from build123d import *

# Parameters (mm, degrees)
SKETCH_1_R          = 12.5
SKETCH_1_R_2        = 3
EXTRUDE_1_DEPTH     = 8
SKETCH_2_R          = 2
CUT_EXTRUDE_1_DEPTH = 13.5
SKETCH_3_R          = 1.5
CUT_EXTRUDE_2_DEPTH = 9.0000001


with BuildPart() as part:
    # 草图1 → 凸台-拉伸1 (new body)
    with BuildSketch(Plane.XY):
        Circle(SKETCH_1_R)
        with Locations((0, -6.3)):
            Circle(SKETCH_1_R_2, mode=Mode.SUBTRACT)
    extrude(amount=EXTRUDE_1_DEPTH)

    # 草图2 → 切除-拉伸1 (cut, through all)
    with BuildSketch(Plane(origin=(0, 0, 0), x_dir=(0, 0, -1), z_dir=(1, 0, 0))):
        with Locations((-4, -6.3)):
            Circle(SKETCH_2_R)
    extrude(amount=-CUT_EXTRUDE_1_DEPTH, mode=Mode.SUBTRACT)

    # 草图3 → 切除-拉伸2 (cut, through all)
    with BuildSketch(Plane.XY.offset(8)):
        with Locations((-5, 5)):
            Circle(SKETCH_3_R)
        with Locations((5, 5)):
            Circle(SKETCH_3_R)
    extrude(amount=-CUT_EXTRUDE_2_DEPTH, mode=Mode.SUBTRACT)


solid = part.part
Design review of the part built by this model. Coordinates are the model's own, in mm. A direction names the side the tool comes from. Coordinates: 2 decimals unless noted, no trailing zeros. Order: outer loops, then holes, each group sorted by start corner. A loop starts at its lowest first (then second) coordinate and runs counter-clockwise, first axis right, second up. Notation, with made-up numbers: M 45,45 L 72,45 A24 cw 72,58 Z; hole C 37.5,-19 d3. An arc over 180 degrees is marked long. Use a Markdown table: item, result.
(1) For faces 1 (the cylindrical face through (-6.2, 4.1, 4.1)), 2 (the cylindrical face through (-6.92, -4.317, 4.26)), list the 3-axis set-ups (+Z, -Z, +X, -X, +Y, -Y) from which the entire face can be reached by the end or side of a thin tool; tool diameter is ignored.
Worked answers:
| item | result |
|---|---|
| face 1 | +Z, -Z |
| face 2 | -X |
(2) Add section D-D (x = 5). Give the boundary of the cut face in (y, z), then the cut area to 3 significant figures.
Worked answers:
| item | result |
|---|---|
| outline | M -11.46,0 L 3.5,0 L 3.5,8 L -11.46,8 Z; M 6.5,0 L 11.46,0 L 11.46,8 L 6.5,8 Z |
| area | 159 mm2 |
(3) Draft analysis for pull direction Y (two halves, no side actions). For faces 3 (the cylindrical face through (11.923, 3.755, 3.944)), 4 (the cylindrical face through (2.86, -5.4, 3.94)), 5 (the flat face through (0, 0, 0)), state which applies: released by +Y, released by -Y, zero draft, split by the parting line, or undercut.
Worked answers:
| item | result |
|---|---|
| face 3 | split by the parting line |
| face 4 | undercut |
| face 5 | zero draft |
(4) Add section C-C (z = 4). Give the boundary of the cut face in (x, y).
Worked answers:
| item | result |
|---|---|
| outline | M -11.74,-4.3 L -2.24,-4.3 A3 cw long -2.24,-8.3 L -9.35,-8.3 A12.5 ccw long Z; hole C -5,5 d3; hole C 5,5 d3 |
(5) Add section B-B (x = 0). Give the boundary of the cut face in (y, z).
Worked answers:
| item | result |
|---|---|
| outline | M -12.5,0 L -9.3,0 L -9.3,8 L -12.5,8 Z; M -3.3,0 L 12.5,0 L 12.5,8 L -3.3,8 Z |
(6) Add section A-A (y = -6.3). Give the boundary of the cut face in (x, z).
Worked answers:
| item | result |
|---|---|
| outline | M -10.8,0 L -3,0 L -3,2 L -10.8,2 Z; M -10.8,6 L -3,6 L -3,8 L -10.8,8 Z; M 3,0 L 10.8,0 L 10.8,8 L 3,8 Z |
(7) For P1, Ø1.5, axis at y = 8, z = 1.5, coming from the -X side; P2, Ø1, axis at x = 7.5, z = 3.5, coming from the -Y side; P3, Ø3, axis at x = 6, z = 2.5, coming from the -Y side, all flat-tipped, find the tip position at first contact; note any pin that passes through.
Worked answers:
| item | result |
|---|---|
| P1 | stops at x = -10.18 |
| P2 | stops at y = -10.36 |
| P3 | stops at y = -11.66 |
(8) Wall thickness on probe 1 along Z at (x, y) = (-6.25, -6.3); probe 2 along X at (y, z) = (-8.75, 7.25); probe 3 along Y at (x, z) = (5, 2): over which ranges is each line inside the solid? List them lowest first.
Worked answers:
| item | result |
|---|---|
| probe 1 | z = 0 to 2, 6 to 8 |
| probe 2 | x = -8.93 to -1.73, 1.73 to 8.93 |
| probe 3 | y = -11.46 to 3.5, 6.5 to 11.46 |
